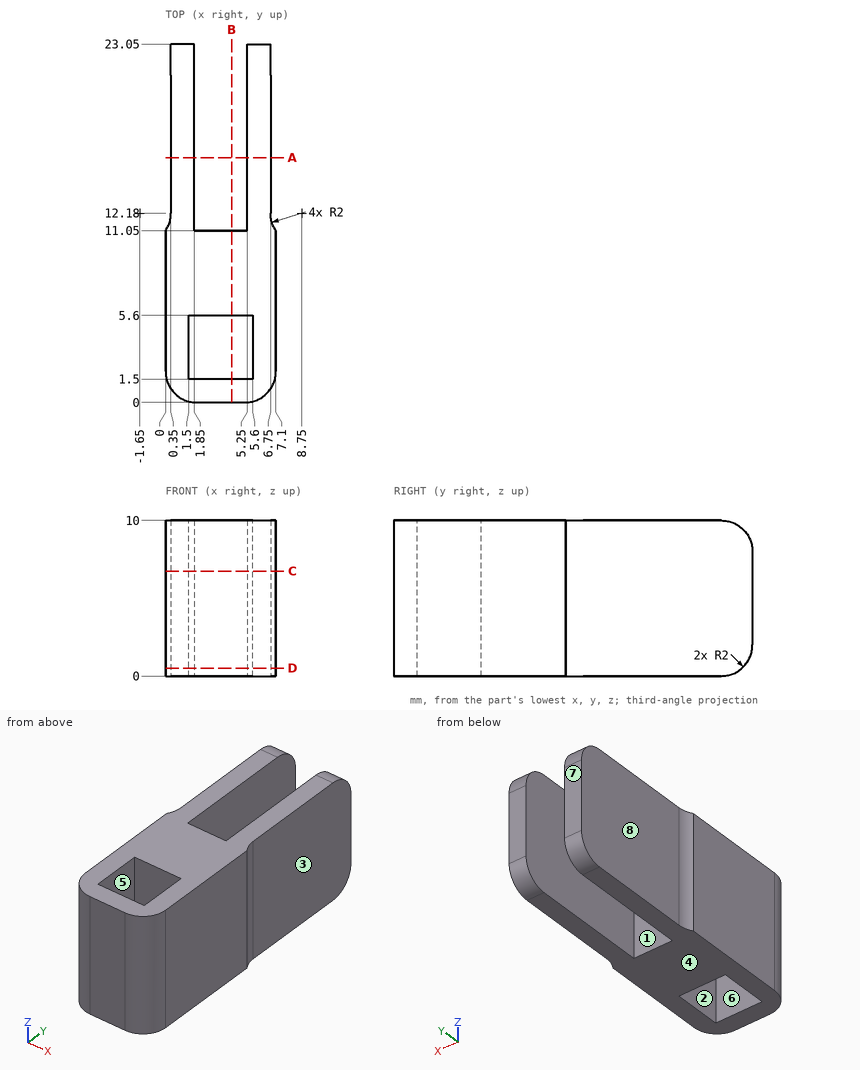
Source: three-view drawing plus pictorial views. Frame: mm from the lowest corner of the part. A direction names the side the tool comes from. Coordinates: 2 decimals unless noted, no trailing zeros. Order: outer loops, then holes, each group sorted by start corner. A loop starts at its lowest first (then second) coordinate and runs counter-clockwise, first axis right, second up. Notation, with made-up numbers: (78.5, -28.75) -> (111.5, -28.75) arc R21 cw to (111.5, -3.75) -> close; hole circle Ø3 at (53.25, -33.5). An arc over 180 degrees is marked (long way). Write item = value, one per line.
(1) Pull-direction query (X, two-part tool) for the marked faces 5, 6, 7 and 8; classes: pulls with the +X half, pulls with the -X half, needs draft (parallel to the pull), parting line crosses it, or undercut.
Solved:
face_5 = undercut
face_6 = undercut
face_7 = needs draft
face_8 = pulls with the -X half
(2) Cut plane A-A on y = 15.75. Return loops of the section in (x, z).
Solved:
outline = (0.35, 0) -> (1.85, 0) -> (1.85, 10) -> (0.35, 10) -> close; (5.25, 0) -> (6.75, 0) -> (6.75, 10) -> (5.25, 10) -> close
(3) Cut plane C-C on z = 6.75. Return loops of the section in (x, y).
Solved:
outline = (0, 2) arc R2 ccw to (2, 0) -> (5.1, 0) arc R2 ccw to (7.1, 2) -> (7.1, 11.05) arc R2 cw to (6.75, 12.18) -> (6.75, 23.05) -> (5.25, 23.05) -> (5.25, 11.05) -> (1.85, 11.05) -> (1.85, 23.05) -> (0.35, 23.05) -> (0.35, 12.18) arc R2 cw to (0, 11.05) -> close; hole (1.5, 1.5) -> (5.6, 1.5) -> (5.6, 5.6) -> (1.5, 5.6) -> close
(4) Line query: line 1 (X direction, y = 4.25, z = 1.5); line 2 (Y direction, x = 2.5, z = 0.75); line 3 (X direction, y = 16, z = 7.5). Output: solid intervals per line, ascending.
Solved:
line_1 = 0 to 1.5, 5.6 to 7.1
line_2 = 0 to 1.5, 5.6 to 11.05
line_3 = 0.35 to 1.85, 5.25 to 6.75
(5) Cut plane B-B on x = 4.25. Return loops of the section in (y, z).
Solved:
outline = (0, 0) -> (1.5, 0) -> (1.5, 10) -> (0, 10) -> close; (5.6, 0) -> (11.05, 0) -> (11.05, 10) -> (5.6, 10) -> close
(6) Access query for the marked faces 1, 2, 3 and 4. Directions: +Z, -Z, +X, -X, +Y, -Y. A direction counts if a zero-diameter tool reaches every point of the face in a straight line with its end or side. Return the directions, or none.
Solved:
face_1 = +Z, -Z, +Y
face_2 = +Z, -Z
face_3 = +Z, -Z, +X, +Y
face_4 = -Z, +X, -X, +Y, -Y
(7) Pin query (flat end, axial travel): pin 1 Ø3 at (y, z) = (16, 5) entering from -X; pin 2 Ø1 at (x, z) = (4.5, 6.5) entering from +Y; pin 3 Ø5 at (y, z) = (16, 1.5) entering from +X. Return the tip coordinate at first contact, or that it passes through.
Solved:
pin_1 = 0.35
pin_2 = 11.05
pin_3 = 6.75
(8) Cut plane D-D on z = 0.5. Return loops of the section in (x, y).
Solved:
outline = (0, 2) arc R2 ccw to (2, 0) -> (5.1, 0) arc R2 ccw to (7.1, 2) -> (7.1, 11.05) arc R2 cw to (6.75, 12.18) -> (6.75, 22.37) -> (5.25, 22.37) -> (5.25, 11.05) -> (1.85, 11.05) -> (1.85, 22.37) -> (0.35, 22.37) -> (0.35, 12.18) arc R2 cw to (0, 11.05) -> close; hole (1.5, 1.5) -> (5.6, 1.5) -> (5.6, 5.6) -> (1.5, 5.6) -> close
